Source: CAD feature listing. Evaluate the final solid. Frame: model axes, mm. A direction names the side the tool comes from. Give positions to 0.01 mm unless a question says otherwise; leave off trailing zeros. Loops run counter-clockwise (first coordinate to the right, second up) from the corner with the lowest first, then second, coordinate; pieces in that order, holes last. Notation, with made-up numbers: M 84.25,19.25 L 129.25,19.25 A13 ccw 129.25,31.25 Z; hole C -13,-31 d9. An arc over 180 degrees is marked long. Put each result on its own line as item: value.
from build123d import *

# Parameters (mm, degrees)
SALIENTE_EXTRUIR1_DEPTH = 7
CROQUIS2_R              = 2.5
CORTAR_EXTRUIR1_DEPTH   = 40
SALIENTE_EXTRUIR2_DEPTH = 6
CORTAR_EXTRUIR2_DEPTH   = 85.364465566
CROQUIS6_R              = 1.5
CORTAR_EXTRUIR3_DEPTH   = 109.399183933
SALIENTE_EXTRUIR3_DEPTH = 2.5
CORTAR_EXTRUIR4_REACH   = 110.399
CROQUIS8_R              = 1.5
CORTAR_EXTRUIR5_REACH   = 84.713
CROQUIS9_R              = 2.5
REDONDEO1_R             = 10


with BuildPart() as part:
    # Croquis1 → Saliente-Extruir1 (new, symmetric)
    with BuildSketch(Plane.XY):
        with BuildLine():
            Line((-73.337453264, -31.996979), (-73.337453264, -16.996979))
            Line((-73.337453264, -16.996979), (-53.337453264, -16.996979))
            Line((-53.337453264, -16.996979), (-33.337453264, -16.996979))
            Line((-33.337453264, -16.996979), (-1.797677202, 7.604698299))
            add(Edge.make_bspline(
                [(-2.271099828, 32.600215317), (-3.120681365, 32.65086638), (-7.140387905, 28.930110418), (-6.851052057, 20.6561771), (-2.970338985, 13.597919356), (-1.149563969, 10.022107474), (-1.797677202, 7.604698299)],
                knots=[0, 0, 0, 0, 0.086865993, 0.573729713, 0.74320117, 1, 1, 1, 1], degree=3))
            add(Edge.make_bspline(
                [(-2.271099828, 32.600215317), (-1.957854214, 32.571324686), (-1.550967765, 32.095962064), (-1.625633045, 30.678221383), (-2.293917384, 28.99060688), (-4.114943029, 21.538574705), (2.702714569, 13.937286445), (10.029738822, 16.830327286)],
                knots=[0, 0, 0, 0, 0.035853338, 0.067043674, 0.168417902, 0.258672943, 1, 1, 1, 1], degree=3))
            Line((10.029738822, 16.830327286), (21.857154848, 26.05595627))
            Line((21.857154848, 26.05595627), (31.082783835, 14.228540246))
            Line((31.082783835, 14.228540246), (-28.179131834, -31.996979))
            Line((-28.179131834, -31.996979), (-73.337453264, -31.996979))
        make_face()
    extrude(amount=SALIENTE_EXTRUIR1_DEPTH, both=True)

    # Croquis2 → Cortar-Extruir1 (cut)
    with BuildSketch(Plane.XY.offset(7)):
        with Locations((-63.337453264, -12.196140351)):
            Circle(CROQUIS2_R)
    extrude(amount=-CORTAR_EXTRUIR1_DEPTH, mode=Mode.SUBTRACT)

    # Croquis4 → Saliente-Extruir2 (add)
    with BuildSketch(Plane.XY.offset(7)):
        Polygon((21.857154848, 26.05595627), (17.914682839, 22.980746608), (27.140311824, 11.153330581), (31.082783835, 14.228540246), align=None)
    saliente_extruir2 = extrude(amount=SALIENTE_EXTRUIR2_DEPTH)

    # Simetría1: Saliente-Extruir2 across plane
    add(saliente_extruir2.mirror(Plane.XY))

    # Croquis5 → Cortar-Extruir2 (cut, through all)
    with BuildSketch(Plane.XY.offset(13)):
        with BuildLine():
            Line((21.227925662, 25.565144498), (21.857154848, 26.05595627))
            Line((21.857154848, 26.05595627), (31.082783835, 14.228540246))
            add(Edge.make_bspline(
                [(31.082783835, 14.228540246), (25.291900343, 19.151696697), (21.227925662, 25.565144498)],
                knots=[0, 0, 0, 1, 1, 1], degree=2))
        make_face()
    extrude(amount=-CORTAR_EXTRUIR2_DEPTH, mode=Mode.SUBTRACT)

    # Croquis6 → Cortar-Extruir3 (cut, through all)
    with BuildSketch(Plane(origin=(22.282654611, 17.3809312, 0), x_dir=(0, 0, 1), z_dir=(-0.7884944017253559, -0.6150419322678522, 0))):
        with Locations((-20.725956244, 4.101908899)):
            Circle(CROQUIS6_R)
        with Locations((-20.725956244, -4.898091102)):
            Circle(CROQUIS6_R)
    cortar_extruir3 = extrude(amount=-CORTAR_EXTRUIR3_DEPTH, mode=Mode.SUBTRACT)

    # Simetría2: Cortar-Extruir3 across plane
    add(cortar_extruir3.mirror(Plane.XY), mode=Mode.SUBTRACT)

    # Croquis7 → Saliente-Extruir3 (add, symmetric)
    with BuildSketch(Plane.XY):
        Polygon((-33.337453264, -16.996979), (-47.567565233, -16.996979), (-63.337565233, -16.996979), (-63.337565233, -9.996979), align=None)
    extrude(amount=SALIENTE_EXTRUIR3_DEPTH, both=True)

    # Croquis8 → Cortar-Extruir4 (cut, up to next)
    with BuildSketch(Plane(origin=(22.282654611, 17.3809312, 0), x_dir=(0, 0, 1), z_dir=(-0.7884944017253558, -0.6150419322678521, 0)), mode=Mode.PRIVATE) as cortar_extruir4_sk1:
        with Locations(Location((-10, 4.479600053, 0), (0, 0, 270))):
            Circle(CROQUIS8_R)
    cortar_extruir4_tool1 = extrude(cortar_extruir4_sk1.sketch, amount=-CORTAR_EXTRUIR4_REACH, mode=Mode.PRIVATE) & part.part
    # Croquis8 → Cortar-Extruir4 (cut, up to next)
    with BuildSketch(Plane(origin=(22.282654611, 17.3809312, 0), x_dir=(0, 0, 1), z_dir=(-0.7884944017253558, -0.6150419322678521, 0)), mode=Mode.PRIVATE) as cortar_extruir4_sk2:
        with Locations(Location((-10, -5.235729918, 0), (0, 0, 270))):
            Circle(CROQUIS8_R)
    cortar_extruir4_tool2 = extrude(cortar_extruir4_sk2.sketch, amount=-CORTAR_EXTRUIR4_REACH, mode=Mode.PRIVATE) & part.part
    cortar_extruir4_1 = cortar_extruir4_tool1.solids().sort_by_distance((19.527513, 20.913071, -10))[0]
    add(cortar_extruir4_1, mode=Mode.SUBTRACT)
    cortar_extruir4_2 = cortar_extruir4_tool2.solids().sort_by_distance((25.502848, 13.252587, -10))[0]
    add(cortar_extruir4_2, mode=Mode.SUBTRACT)
    cortar_extruir4 = cortar_extruir4_1 + cortar_extruir4_2  # Cortar-Extruir4 as one shape, for the pattern or mirror that repeats it

    # Simetría3: Cortar-Extruir4 across plane
    add(cortar_extruir4.mirror(Plane.XY), mode=Mode.SUBTRACT)

    # Croquis9 → Cortar-Extruir5 (cut, up to next)
    with BuildSketch(Plane.XY.offset(7), mode=Mode.PRIVATE) as cortar_extruir5_sk1:
        with Locations((-63.337453264, -24.496979)):
            Circle(CROQUIS9_R)
    cortar_extruir5_tool1 = extrude(cortar_extruir5_sk1.sketch, amount=-CORTAR_EXTRUIR5_REACH, mode=Mode.PRIVATE) & part.part
    add(cortar_extruir5_tool1.solids().sort_by_distance((-63.337453, -24.496979, 7))[0], mode=Mode.SUBTRACT)

    # Redondeo1
    # the kernel refuses this fillet: 10 mm, written as the material it takes off along each edge
    with BuildSketch(Plane(origin=(-73.337453264, -16.996979, 32), x_dir=(0, -1, 0), z_dir=(0, 0, -1))) as redondeo1_piece_1:
        with BuildLine():
            CenterArc((REDONDEO1_R, -REDONDEO1_R), REDONDEO1_R, 90, 90)
            Line((0, -REDONDEO1_R), (0, 0))
            Line((0, 0), (REDONDEO1_R, 0))
        make_face()
    extrude(amount=64, mode=Mode.SUBTRACT)


solid = part.part
1. Draft query along Z for faces 1 (the flat face through (-19, -9, 7)), 2 (the cylindrical face through (-70.486, -20.004, 0.098)), 3 (the cylindrical face through (28.239, 13.572, 9.549)), 4 (the flat face through (-55, -15, -2.5)). Return one class per face: pulls with the +Z half, pulls with the -Z half, needs draft (parallel to the pull), parting line crosses it, or undercut.
Found:
face 1: pulls with the +Z half
face 2: needs draft
face 3: undercut
face 4: pulls with the -Z half
2. Section query B-B (y = 3.5). Output: boundary loops of the cut face in (x, z).
Found:
outline: M -7.06,-7 L 17.33,-7 L 17.33,7 L -7.06,7 Z
3. Section query A-A (x = -42.5). Output: boundary loops of the cut face in (y, z), plus the area to 3 significant figures.
Found:
outline: M -32,-7 L -17,-7 L -17,-2.5 L -14.86,-2.5 L -14.86,2.5 L -17,2.5 L -17,7 L -32,7 Z
area: 221 mm^2
4. Contact query for flat-ended pins moving along their axis: P1, Ø10, axis at x = -62, z = 0, coming from the +Y side; P2, Ø10, axis at x = -9, y = -6, coming from the +Z side; P3, Ø5, axis at x = -49.5, z = 3.5, coming from the +Y side. Output: stop coordinate, or through.
Found:
P1: y = -10
P2: z = 7
P3: y = -12.69
5. Access query for faces 5 (the flat face through (22.5, 17.1, -10)), 6 (the flat face through (-63.338, -14, 0)), 7 (the flat face through (-55, -15, 2.5)). Directions: +Z, -Z, +X, -X, +Y, -Y. A direction counts if a zero-diameter tool reaches every point of the face in a straight line with its end or side. Return the directions, or none.
Found:
face 5: -Z, -X, -Y
face 6: +Z, -Z, -X, +Y
face 7: +Z, -X, +Y
6. Material intervals for line 1 (Y direction, x = -34, z = -3.5); line 2 (Z direction, x = -51.5, y = -18); line 3 (Y direction, x = -3, z = -6.25), sorted ascending. Write a range as from..to.
Found:
line 1: -32..-17
line 2: -7..7
line 3: -12.36..6.67, 13.58..32.49
7. Section query D-D (y = -20). Output: boundary loops of the cut face in (x, z).
Found:
outline: M -70.48,-7 L -12.8,-7 L -12.8,7 L -70.48,7 Z
8. Section query C-C (x = -59). Output: boundary loops of the cut face in (y, z).
Found:
outline: M -32,-7 L -17,-7 L -17,-2.5 L -11.01,-2.5 L -11.01,2.5 L -17,2.5 L -17,7 L -32,7 Z
